Geometry: final body of the model. Coordinates: model frame, mm. A direction names the side the tool comes from. Give positions to 0.01 mm unless a question says otherwise; leave off trailing zeros. Write each loop counter-clockwise with the first axis right and the second up, starting at its lowest first coordinate (ties: lowest second). Pieces come first, ordered by that corner, then holes.
Q1. Reachability of faces 4 (the flat face through (18, 1, 4.48)), 5 (the flat face through (18, 0, 4)) from +Z, -Z, +X, -X, +Y, -Y: full face, straight path, thin tool, end or side. Return the list, or none.
Q2. Line query: line 1 (Y direction, x = 13, z = 5); line 2 (Z direction, x = 29, y = 45); line 3 (X direction, y = 6, z = 7.5). Output: solid intervals per line, ascending.
Q3. Section C-C (x = 4.5). Return the cut outline in (y, z) (3 decimals), plus the area to 3 significant figures.
Q4. Section B-B (y = 65.5). Return the cut outline in (x, z) (3 decimals), plus the area to 3 significant figures.
Q5. Section A-A (z = 7.25). Return the cut outline in (x, y), plus the area to 3 significant figures.
Q6. Section D-D (x = 20.5). Return the cut outline in (y, z) (3 decimals).
Q7. Pin query (flat end, axial travel): pin 1 Ø12 at (x, y) = (19, 38.5) entering from +Z; pin 2 Ø3 at (y, z) = (3.38, 5.03) entering from +X; pin 3 Ø1.9 at (x, y) = (18, 1.5) entering from +Z; pin 4 Ø1.5 at (y, z) = (67, 7) entering from +X. Return the tip coordinate at first contact, or that it passes through.
Q8. Mould query, pull axis X, two halves, no side actions, for faces 1 (the flat face through (23.23, 42.4, 6.34)), 2 (the cylindrical face through (34.549, 42.398, 2.324)), 3 (the flat face through (30, 42, 8.15)). Classes: +X half, -X half, draft (parallel to the pull), parting line (faces both ways), or undercut.
Autodesk Fusion 360 part; units mm, degrees
sketch "Sketch1" plane through (0, 0, 0) normal (0, 1, 0) x (1, 0, 0)
  line L0 (0, 0) -> (37, 0)
  line L1 (37, 0) -> (37, -8.15)
  line L2 (37, -8.15) -> (0, -8.15)
  line L3 (0, -8.15) -> (0, 0)
  line L4 (37, -8.15) -> (28.85, -8.15)
  line L5 (28.85, -8.15) -> (28.85, 0)
  line L6 (28.85, 0) -> (37, 0)
  line L7 (37, 0) -> (37, -8.15)
  arc A0 (37, -8.15) -> (28.85, 0) centre (28.85, -8.15) ccw
  line L8 (0, -8.15) -> (8.15, -8.15)
  line L9 (8.15, -8.15) -> (8.15, 0)
  line L10 (8.15, 0) -> (0, 0)
  line L11 (0, 0) -> (0, -8.15)
  arc A1 (8.15, 0) -> (0, -8.15) centre (8.15, -8.15) ccw
  dimension "d1" = 37
  dimension "d2" = 8.15
  dimension "d3" = 8.15
  dimension "d4" = 8.15
  dimension "d5" = 8.15
  dimension "d6" = 8.15
extrude "Extrude1" add sketch "Sketch1" along normal blind 86 contours L0 L2 L5 L9 | L2 L8 L9 A1 | L2 L4 L5 A0
sketch "Sketch2" plane through (0, 0, 0) normal (0, -1, 0) x (1, 0, 0)
  arc A0 (28.85, 0) -> (37, 8.15) centre (28.85, 8.15) ccw
  line L0 (37, 8.15) -> (0, 8.15)
  arc A1 (0, 8.15) -> (8.15, 0) centre (8.15, 8.15) ccw
  line L1 (8.15, 0) -> (28.85, 0)
  line L2 (18.5, 8.15) -> (18.5, 0)
  line L3 (13.125, 4.48) -> (23.875, 4.48)
  line L4 (14.4, 8.15) -> (22.6, 8.15)
  line L5 (14.4, 8.15) -> (13.125, 4.48)
  line L6 (22.6, 8.15) -> (23.875, 4.48)
  dimension "d9" = 10.75
  dimension "d10" = 3.67
  dimension "d11" = 8.2
extrude "Extrude2" cut sketch "Sketch2" against normal blind 115 contours L0 L2 L3 L4 L6 | L0 L2 L3 L4 L5
sketch "Sketch3" plane through (0, 0, 0) normal (1, 0, 0) x (0, 1, 0)
  circle A0 centre (3.3767, 5.025) radius 1.125
  line L0 (-5, 8) -> (-5, 0)
  line L1 (-3.6483, 8.15) -> (5, 8.15)
  line L2 (5, 8.15) -> (5, -1.85)
  line L3 (5, -1.85) -> (-3.6483, -1.85)
  line L4 (-3.6483, -1.85) -> (-3.6483, 8.15)
  line L5 (0, 8.15) -> (86, 8.15)
  dimension "d14" = 2.25
  dimension "d16" = 5.9
  dimension "d17" = 2
extrude "Extrude3" cut sketch "Sketch3" along normal blind 48 contours A0
Computed:
1. face 4: +Y, -Y
1. face 5: +Z, -Z, +X, -X, -Y
2. line 1: y = 0 to 2.25, 4.5 to 86
2. line 2: z = 0 to 8.15
2. line 3: x = 0.03 to 14.17, 22.83 to 36.97
3. outline: (0, 0.863) - (86, 0.863) - (86, 8.15) - (0, 8.15) - close; hole circle Ø2.25 at (3.377, 5.025)
3. area: 623 mm2
4. outline: (0, 8.15) arc R8.15 ccw to (8.15, 0) - (28.85, 0) arc R8.15 ccw to (37, 8.15) - (22.6, 8.15) - (23.875, 4.48) - (13.125, 4.48) - (14.4, 8.15) - close
4. area: 238 mm2
5. outline: (0.05, 0) - (14.09, 0) - (14.09, 86) - (0.05, 86) - close; (22.91, 0) - (36.95, 0) - (36.95, 86) - (22.91, 86) - close
5. area: 2,410 mm2
6. outline: (0, 0) - (86, 0) - (86, 4.48) - (4.361, 4.48) arc R1.125 cw to (2.393, 4.48) - (0, 4.48) - close
7. pin 1: stops at z = 8.15
7. pin 2: stops at x = 36.84
7. pin 3: stops at z = 4.48
7. pin 4: stops at x = 36.99
8. face 1: undercut
8. face 2: +X half
8. face 3: draft
